from build123d import *

# Parameters (mm, degrees)
SKETCH3_W           = 20
SKETCH3_H           = 20
BOSS_EXTRUDE1_DEPTH = 1.5
SKETCH4_R           = 1.5
BOSS_EXTRUDE2_DEPTH = 1.5
SKETCH5_R           = 1
SKETCH5_R_2         = 2.5
CUT_EXTRUDE1_DEPTH  = 1.5
SKETCH6_W           = 5
SKETCH6_H           = 10
BOSS_EXTRUDE3_DEPTH = 8
SKETCH7_R           = 6
BOSS_EXTRUDE4_DEPTH = 7
FILLET1_R           = 0.5
SKETCH8_R           = 1.5
CUT_EXTRUDE2_DEPTH  = 3


with BuildPart() as part:
    # Sketch3 → Boss-Extrude1 (new body)
    with BuildSketch(Plane(origin=(0, 0, 0), x_dir=(1, 0, 0), z_dir=(0, 1, 0))):
        Rectangle(SKETCH3_W, SKETCH3_H)
    extrude(amount=BOSS_EXTRUDE1_DEPTH)

    # Sketch4 → Boss-Extrude2 (add)
    with BuildSketch(Plane(origin=(0, 1.5, 0), x_dir=(1, 0, 0), z_dir=(0, 1, 0))):
        with Locations((-10, 0)):
            Circle(SKETCH4_R)
        with Locations((10, 0)):
            Circle(SKETCH4_R)
    extrude(amount=-BOSS_EXTRUDE2_DEPTH)

    # Sketch5 → Cut-Extrude1 (cut)
    with BuildSketch(Plane(origin=(0, 1.5, 0), x_dir=(1, 0, 0), z_dir=(0, 1, 0))):
        with Locations((-10, 0)):
            Circle(SKETCH5_R)
        with Locations((10, 0)):
            Circle(SKETCH5_R)
        with Locations((0, 10)):
            Circle(SKETCH5_R_2)
        with Locations((0, -10)):
            Circle(SKETCH5_R_2)
    extrude(amount=-CUT_EXTRUDE1_DEPTH, mode=Mode.SUBTRACT)

    # Sketch6 → Boss-Extrude3 (add)
    with BuildSketch(Plane(origin=(0, 1.5, 0), x_dir=(1, 0, 0), z_dir=(0, 1, 0))):
        with Locations((-6.006775527, 0)):
            Rectangle(SKETCH6_W, SKETCH6_H)
    extrude(amount=BOSS_EXTRUDE3_DEPTH)

    # Sketch7 → Boss-Extrude4 (add)
    with BuildSketch(Plane(origin=(0, 1.5, 0), x_dir=(1, 0, 0), z_dir=(0, 1, 0))):
        with Locations((2.7, 0)):
            Circle(SKETCH7_R)
    extrude(amount=BOSS_EXTRUDE4_DEPTH)

    # Fillet1
    fillet1_edges = [part.edges().sort_by_distance(p)[0] for p in [
        (-3.3, 8.5, 0),
    ]]
    fillet(fillet1_edges, radius=FILLET1_R)

    # Sketch8 → Cut-Extrude2 (cut)
    with BuildSketch(Plane(origin=(0, 8.5, 0), x_dir=(1, 0, 0), z_dir=(0, 1, 0))):
        with Locations((2.7, 0)):
            Circle(SKETCH8_R)
    extrude(amount=-CUT_EXTRUDE2_DEPTH, mode=Mode.SUBTRACT)


solid = part.part
Part model, mm, in its own coordinate system. A direction names the side the tool comes from. Coordinates: 2 decimals unless noted, no trailing zeros. Write each loop counter-clockwise with the first axis right and the second up, starting at its lowest first coordinate (ties: lowest second). Pieces come first, ordered by that corner, then holes. Notation, with made-up numbers: (67.5, 31.5) - (71.5, 31.5) arc R21 ccw to (71.5, 56.5) - close; hole circle Ø4 at (26.25, -20). An arc over 180 degrees is marked (long way). Put each result on its own line as item: value.
1. Probe line 1 along X through (y, z) = (7.7, 0); line 2 along X through (y, z) = (0.55, 0); line 3 along Z through (x, y) = (2.7, 6.4). List the from-to ranges inside material, lowest first. Write a range as [from, to].
Final values:
line 1: x = [-8.51, -3.51], [-3.3, 1.2], [4.2, 8.7]
line 2: x = [-11.5, -11], [-9, 9], [11, 11.5]
line 3: z = [-6, -1.5], [1.5, 6]
2. Flat gauge pins, fed straight in: pin 1 Ø0.8 at (y, z) = (1, -5) entering from -X; pin 2 Ø3.5 at (x, z) = (2.5, 0) entering from +Y; pin 3 Ø4 at (x, y) = (0, 4.5) entering from +Z; pin 4 Ø1.5 at (x, z) = (-3.5, 7.5) entering from -Y. Where does each tip first touch, or does it go through?
Final values:
pin 1: stops at x = -10
pin 2: stops at y = 8.5
pin 3: stops at z = 5.96
pin 4: stops at y = 0
3. Band-saw the part on B-B (x = -5.25). Write the cut outline in (y, z), then the cut area to 3 significant figures.
Final values:
outline: (0, -10) - (1.5, -10) - (1.5, -5) - (9.5, -5) - (9.5, 5) - (1.5, 5) - (1.5, 10) - (0, 10) - close
area: 110 mm²
4. Band-saw the part on C-C (y = 1). Write the cut outline in (x, z).
Final values:
outline: (-10, -10) - (-2.5, -10) arc R2.5 cw to (2.5, -10) - (10, -10) - (10, -1.5) arc R1.5 ccw to (10, 1.5) - (10, 10) - (2.5, 10) arc R2.5 cw to (-2.5, 10) - (-10, 10) - (-10, 1.5) arc R1.5 ccw to (-10, -1.5) - close; hole circle Ø2 at (-10, 0); hole circle Ø2 at (10, 0)
5. Two-plate mould, pull along X, no slides. Class faces 5 (the flat face through (-10, 1, -6)), 6 (the cylindrical face through (-2.06, 4.7, 3.65)), 7 (the flat face through (6, 1, 10)): +X half, -X half, draft (parallel to the pull), parting line (faces both ways), or undercut.
Final values:
face 5: -X half
face 6: undercut
face 7: draft
6. Band-saw the part on A-A (z = 0). Write the cut outline in (x, y), then the cut area to 3 significant figures.
Final values:
outline: (-11.5, 0) - (-11, 0) - (-11, 1.5) - (-11.5, 1.5) - close; (-9, 0) - (9, 0) - (9, 1.5) - (8.7, 1.5) - (8.7, 8) arc R0.5 ccw to (8.2, 8.5) - (4.2, 8.5) - (4.2, 5.5) - (1.2, 5.5) - (1.2, 8.5) - (-2.8, 8.5) arc R0.5 ccw to (-3.3, 8) - (-3.3, 1.5) - (-3.51, 1.5) - (-3.51, 9.5) - (-8.51, 9.5) - (-8.51, 1.5) - (-9, 1.5) - close; (11, 0) - (11.5, 0) - (11.5, 1.5) - (11, 1.5) - close
area: 143 mm²
7. 3-axis set-ups, long thin cutter, end or side, ignore diameter. For faces 1 (the flat face through (-6, 5, -5)), 2 (the flat face through (-10, 1, 6)), 3 (the flat face through (3, 5.5, 0)), 4 (the flat face through (10, 1, 6)): which of +Z, -Z, +X, -X, +Y, -Y reach the whole face in a straight line?
Final values:
face 1: -Z, -X, +Y
face 2: +Z, -X, +Y, -Y
face 3: +Y
face 4: +Z, +X, +Y, -Y
